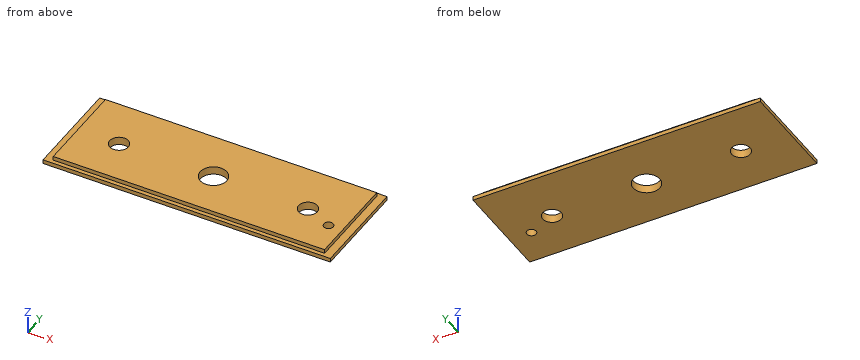
```python
from build123d import *

# Parameters (mm, degrees)
SKETCH_W        = 108
SKETCH_H        = 38
PAD_DEPTH       = 3
SKETCH002_W     = 3
SKETCH002_H     = 38
POCKET_DEPTH    = 1.5
SKETCH003_W     = 3
SKETCH003_H     = 38
POCKET001_DEPTH = 1.5
SKETCH004_W     = 102
SKETCH004_H     = 1.5
POCKET002_DEPTH = 1.5
SKETCH005_W     = 102
SKETCH005_H     = 1.5
POCKET003_DEPTH = 1.5
SKETCH006_R     = 5
POCKET004_DEPTH = 3
SKETCH008_R     = 3.5
POCKET005_DEPTH = 3
SKETCH009_R     = 3.5
POCKET006_DEPTH = 3
SKETCH010_R     = 1.75
POCKET007_DEPTH = 3


with BuildPart() as part:
    # Sketch → Pad (new body)
    with BuildSketch(Plane.XY):
        with Locations((54, -19)):
            Rectangle(SKETCH_W, SKETCH_H)
    extrude(amount=PAD_DEPTH)

    # Sketch002 (on Face6 of Pad) → Pocket (cut)
    with BuildSketch(Plane.XY.offset(3)):
        with Locations((1.5, -19)):
            Rectangle(SKETCH002_W, SKETCH002_H)
    extrude(amount=-POCKET_DEPTH, mode=Mode.SUBTRACT)

    # Sketch003 (on Face4 of Pocket) → Pocket001 (cut)
    with BuildSketch(Plane.XY.offset(3)):
        with Locations((106.5, -19)):
            Rectangle(SKETCH003_W, SKETCH003_H)
    extrude(amount=-POCKET001_DEPTH, mode=Mode.SUBTRACT)

    # Sketch004 (on Face6 of Pocket001) → Pocket002 (cut)
    with BuildSketch(Plane.XY.offset(3)):
        with Locations((54, -0.75)):
            Rectangle(SKETCH004_W, SKETCH004_H)
    extrude(amount=-POCKET002_DEPTH, mode=Mode.SUBTRACT)

    # Sketch005 (on Face12 of Pocket002) → Pocket003 (cut)
    with BuildSketch(Plane.XY.offset(3)):
        with Locations((54, -37.25)):
            Rectangle(SKETCH005_W, SKETCH005_H)
    extrude(amount=-POCKET003_DEPTH, mode=Mode.SUBTRACT)

    # Sketch006 (on Face13 of Pocket003) → Pocket004 (cut)
    with BuildSketch(Plane.XY.offset(3)):
        with Locations((54, -20)):
            Circle(SKETCH006_R)
    extrude(amount=-POCKET004_DEPTH, mode=Mode.SUBTRACT)

    # Sketch008 (on Face14 of Pocket004) → Pocket005 (cut)
    with BuildSketch(Plane.XY.offset(3)):
        with Locations((18.5, -20)):
            Circle(SKETCH008_R)
    extrude(amount=-POCKET005_DEPTH, mode=Mode.SUBTRACT)

    # Sketch009 (on Face15 of Pocket005) → Pocket006 (cut)
    with BuildSketch(Plane.XY.offset(3)):
        with Locations((89.5, -20)):
            Circle(SKETCH009_R)
    extrude(amount=-POCKET006_DEPTH, mode=Mode.SUBTRACT)

    # Sketch010 (on Face16 of Pocket006) → Pocket007 (cut)
    with BuildSketch(Plane.XY.offset(3)):
        with Locations((99.75, -24.5)):
            Circle(SKETCH010_R)
    extrude(amount=-POCKET007_DEPTH, mode=Mode.SUBTRACT)


solid = part.part
```
Geometry check sheet. Reference: the model listing, model coordinates, mm. Round coordinates to 2 decimals unless told otherwise and drop trailing zeros. Order: outer loops, then holes, each group sorted by start corner. A loop starts at its lowest first (then second) coordinate and runs counter-clockwise, first axis right, second up. Notation, with made-up numbers: M 11.5,63.5 L 34.5,63.5 A13 ccw 34.5,80.5 Z; hole C 10.5,40 d4. An arc over 180 degrees is marked long. Write item = value, one per line.
Q1. Section check A-A (x = 54). Enter the section's corners in (y, z).
Answer block:
outline = M -38,0 L -25,0 L -25,3 L -36.5,3 L -36.5,1.5 L -38,1.5 Z; M -15,0 L 0,0 L 0,1.5 L -1.5,1.5 L -1.5,3 L -15,3 Z
Q2. Section check B-B (y = -18). Enter the section's corners in (x, z).
Answer block:
outline = M 0,0 L 15.63,0 L 15.63,3 L 3,3 L 3,1.5 L 0,1.5 Z; M 21.37,0 L 49.42,0 L 49.42,3 L 21.37,3 Z; M 58.58,0 L 86.63,0 L 86.63,3 L 58.58,3 Z; M 92.37,0 L 108,0 L 108,1.5 L 105,1.5 L 105,3 L 92.37,3 Z
Q3. Section check D-D (y = -6). Enter the section's corners in (x, z), plus the area to 3 significant figures.
Answer block:
outline = M 0,0 L 108,0 L 108,1.5 L 105,1.5 L 105,3 L 3,3 L 3,1.5 L 0,1.5 Z
area = 315 mm^2
Q4. Depth check by flat-ended pin: pin 1 Ø2 at (x, y) = (99.75, -24.5) entering from -Z; pin 2 Ø0.8 at (x, z) = (50, 2) entering from +Y; pin 3 Ø0.8 at (y, z) = (-26.5, 2) entering from +X. Enter the tip coordinate at first touch or a pass-through.
Answer block:
pin_1 = through
pin_2 = -1.5
pin_3 = 105
Q5. Scan lines: line 1 (X direction, y = -17, z = 2.65); line 2 (Y direction, x = 54, z = 0.9); line 3 (Y direction, x = 89.5, z = 1.3). Record each from-to range of solid material in increasing order.
Answer block:
line_1 = 3 to 16.7, 20.3 to 50, 58 to 87.7, 91.3 to 105
line_2 = -38 to -25, -15 to 0
line_3 = -38 to -23.5, -16.5 to 0
Q6. Section check C-C (z = 2.3). Enter the section's corners in (x, y), plus the area to 3 significant figures.
Answer block:
outline = M 3,-36.5 L 105,-36.5 L 105,-1.5 L 3,-1.5 Z; hole C 18.5,-20 d7; hole C 54,-20 d10; hole C 89.5,-20 d7; hole C 99.75,-24.5 d3.5
area = 3,400 mm^2
